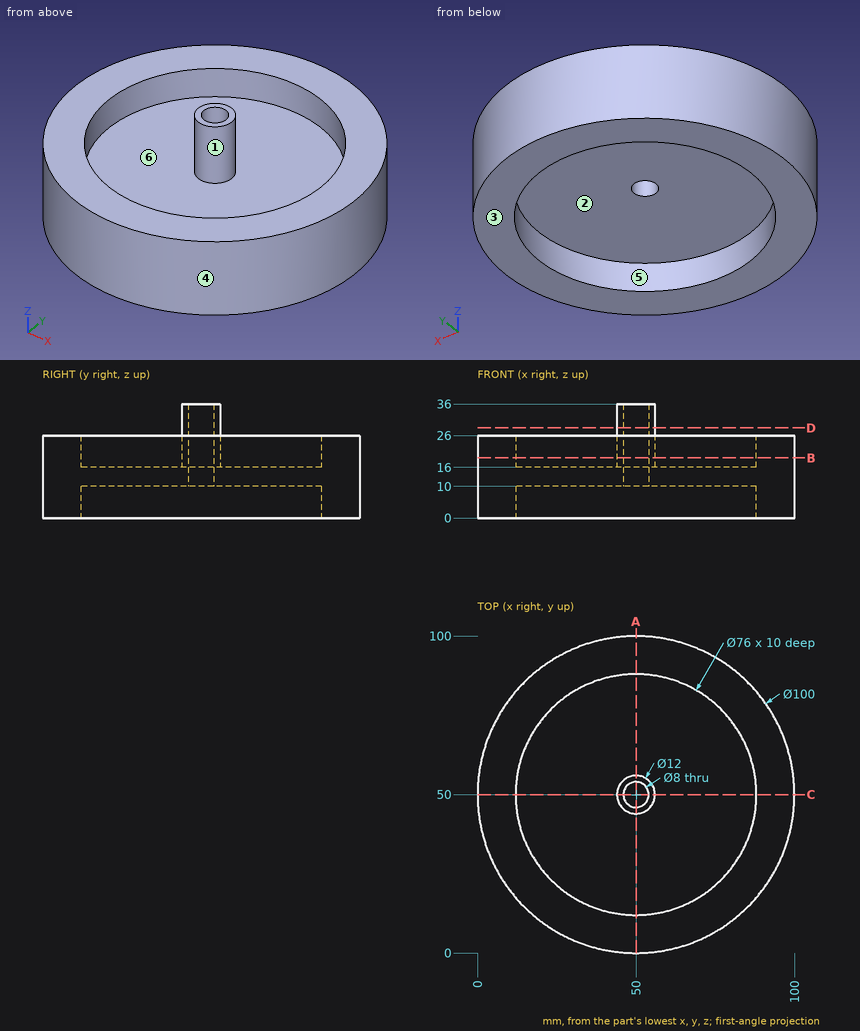
Geometry: see drawing. Coordinates: mm, zero at the bounding-box minimum. A direction names the side the tool comes from. Round coordinates to 2 decimals unless told otherwise and drop trailing zeros. Write each loop counter-clockwise with the first axis right and the second up, starting at its lowest first coordinate (ties: lowest second). Pieces come first, ordered by that corner, then holes.
1) Cut plane B-B (z = 19). Return the cut outline in (x, y).
2) Cut plane D-D (z = 28.5). Return the cut outline in (x, y).
3) Ray query, L1, parallel to Y at x = 50, z = 18; L2, parallel to Y at x = 50, z = 2.75; L3, parallel to Y at x = 45, z = 17. Return the intervals inside material, ascending.
4) Cut plane A-A (x = 50). Return the cut outline in (y, z), then the cut area to 3 significant figures.
5) Draft query along X for the marked faces 3, 4, 5 and 6. Return one class per face: pulls with the +X half, pulls with the -X half, needs draft (parallel to the pull), parting line crosses it, or undercut.
6) Reachability of the marked faces 1 and 2 from +Z, -Z, +X, -X, +Y, -Y: full face, straight path, thin tool, end or side. Return the list, or none.
7) Contact query for flat-ended pins moving along their axis: P1, Ø6, axis at y = 70, z = 29.5, coming from the +X side; P2, Ø8, axis at x = 51, z = 25.5, coming from the +Y side; P3, Ø4, axis at x = 78.5, y = 60, coming from the -Z side; P4, Ø23, axis at x = 67, y = 53, coming from the +Z side. Output: stop coordinate, or through.
Geometry says:
1. outline: circle Ø100 at (50, 50); circle Ø12 at (50, 50); hole circle Ø76 at (50, 50); hole circle Ø8 at (50, 50)
2. outline: circle Ø12 at (50, 50); hole circle Ø8 at (50, 50)
3. L1: y = 0 to 12, 44 to 46, 54 to 56, 88 to 100
3. L2: y = 0 to 12, 88 to 100
3. L3: y = 0.25 to 12.33, 46.68 to 53.32, 87.67 to 99.75
4. outline: (0, 0) - (12, 0) - (12, 10) - (46, 10) - (46, 36) - (44, 36) - (44, 16) - (12, 16) - (12, 26) - (0, 26) - close; (54, 10) - (88, 10) - (88, 0) - (100, 0) - (100, 26) - (88, 26) - (88, 16) - (56, 16) - (56, 36) - (54, 36) - close
4. area: 1,110 mm2
5. face 3: needs draft
5. face 4: parting line crosses it
5. face 5: undercut
5. face 6: undercut
6. face 1: +Z
6. face 2: -Z
7. P1: passes through
7. P2: stops at y = 100
7. P3: stops at z = 10
7. P4: stops at z = 36
